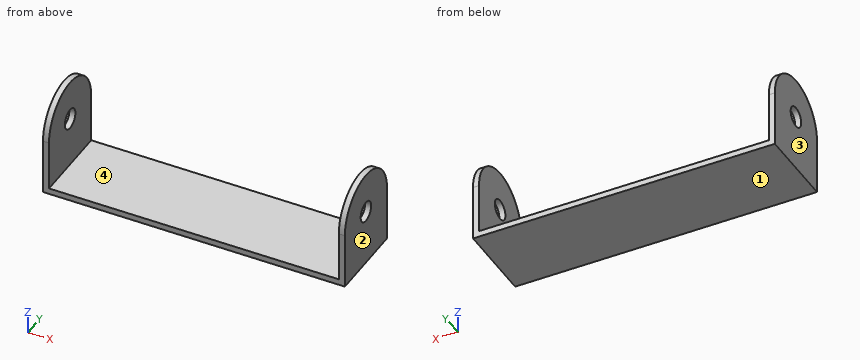
Autodesk Inventor part; units mm, degrees
ref_plane "YZ Plane" through (0, 0, 0) normal (1, 0, 0) x (0, 1, 0)
ref_plane "XZ Plane" through (0, 0, 0) normal (0, 1, 0) x (-1, 0, 0)
ref_plane "XY Plane" through (0, 0, 0) normal (0, 0, 1) x (1, 0, 0)
sketch "스케치1" plane through (0, 0, 0) normal (0, 0, 1) x (1, 0, 0)
  line L0 (0, 0) -> (150, 0)
  line L1 (150, 0) -> (150, 40)
  line L2 (150, 40) -> (0, 40)
  line L3 (0, 40) -> (0, 0)
  point P0 (150, 20)
  dimension "d0" = 40
  dimension "d1" = 150
extrude "돌출1" add sketch "스케치1" along normal blind 3
sketch "스케치2" plane through (0, 0, 0) normal (-1, 0, 0) x (0, 0, 1)
  line L0 (3, 0) -> (3, 40)
  line L1 (3, 40) -> (28, 40)
  line L2 (28, 0) -> (3, 0)
  line L3 (3, 0) -> (3, 40)
  arc A0 (28, 0) -> (28, 40) centre (28, 20) ccw
  circle A1 centre (28, 20) radius 5
  point P0 (0, 0)
  dimension "d5" = 10
  dimension "d6" = 25
extrude "돌출2" add sketch "스케치2" against normal blind 3
sketch "스케치3" plane through (150, 0, 0) normal (1, 0, 0) x (0, 0, -1)
  line L0 (-3, 0) -> (-3, 40)
  arc A0 (-28, 40) -> (-28, 0) centre (-28, 20) ccw
  line L1 (-3, 0) -> (-28, 0)
  line L2 (0, 40) -> (-28, 40)
  line L3 (-28, 40) -> (-3, 40)
  arc A1 (-28, 40) -> (-28, 0) centre (-28, 20) ccw
  circle A2 centre (-28, 20) radius 5
  circle A3 centre (-28, 20) radius 5
  point P0 (0, 0)
  dimension "d10" = 10
extrude "돌출3" add sketch "스케치3" against normal blind 3
properties part number "braket"
Could you check a few things on this model? Use its own coordinates, in mm. Face numbers are marked on the shaded views. Give positions to 0.01 mm unless a question says otherwise; leave off trailing zeros. Loops run counter-clockwise (first coordinate to the right, second up) from the corner with the lowest first, then second, coordinate; pieces in that order, holes last. Notation, with made-up numbers: M 7,30.25 L 45,30.25 A17 cw 45,37.25 Z; hole C 24,-14 d2. An arc over 180 degrees is marked long. Answer as a JSON object with one key per item and string values.
Q1. Suppose I cut it at B-B, the plane y = 20. List the corners of the cut face in (x, z) for me.
Values found:
{"outline": "M 0,0 L 150,0 L 150,23 L 147,23 L 147,3 L 3,3 L 3,23 L 0,23 Z; M 0,33 L 3,33 L 3,48 L 0,48 Z; M 147,33 L 150,33 L 150,48 L 147,48 Z"}
Q2. Suppose I cut it at C-C, the plane x = 44.5. List the corners of the cut face in (y, z) for me, plus the area to 3 significant figures.
Values found:
{"outline": "M 0,0 L 40,0 L 40,3 L 0,3 Z", "area": "120 mm²"}
Q3. If we mould it in two halves opening along X, with no side actions, what happens to the marked faces 1, 2, 3 and 4? For each: pulls with the +X half, pulls with the -X half, needs draft (parallel to the pull), parting line crosses it, or undercut.
Values found:
{"face 1": "needs draft", "face 2": "pulls with the +X half", "face 3": "pulls with the -X half", "face 4": "undercut"}
Q4. For P1, Ø8, axis at y = 20, z = 28, coming from the +X side; P2, Ø12, axis at x = 71, y = 14, coming from the +Z side, each with a flat end and sliding along its axis, tell me the tip position at first contact or that it passes through.
Values found:
{"P1": "passes through", "P2": "stops at z = 3"}
Q5. Suppose I cut it at D-D, the plane y = 33. List the corners of the cut face in (x, z) for me.
Values found:
{"outline": "M 0,0 L 150,0 L 150,43.2 L 147,43.2 L 147,3 L 3,3 L 3,43.2 L 0,43.2 Z"}
Q6. If I drill on probe 1 along X at (y, z) = (32.5, 40); probe 2 along Y at (x, z) = (2, 28); probe 3 along Z at (x, y) = (126, 8), over which ranges is the centre line in solid material (lowest first)? Write a range as [from, to].
Values found:
{"probe 1": "x = [0, 3], [147, 150]", "probe 2": "y = [0, 15], [25, 40]", "probe 3": "z = [0, 3]"}
Q7. Suppose I cut it at A-A, the plane z = 15.5. List the corners of the cut face in (x, y) for me.
Values found:
{"outline": "M 0,0 L 3,0 L 3,40 L 0,40 Z; M 147,0 L 150,0 L 150,40 L 147,40 Z"}
